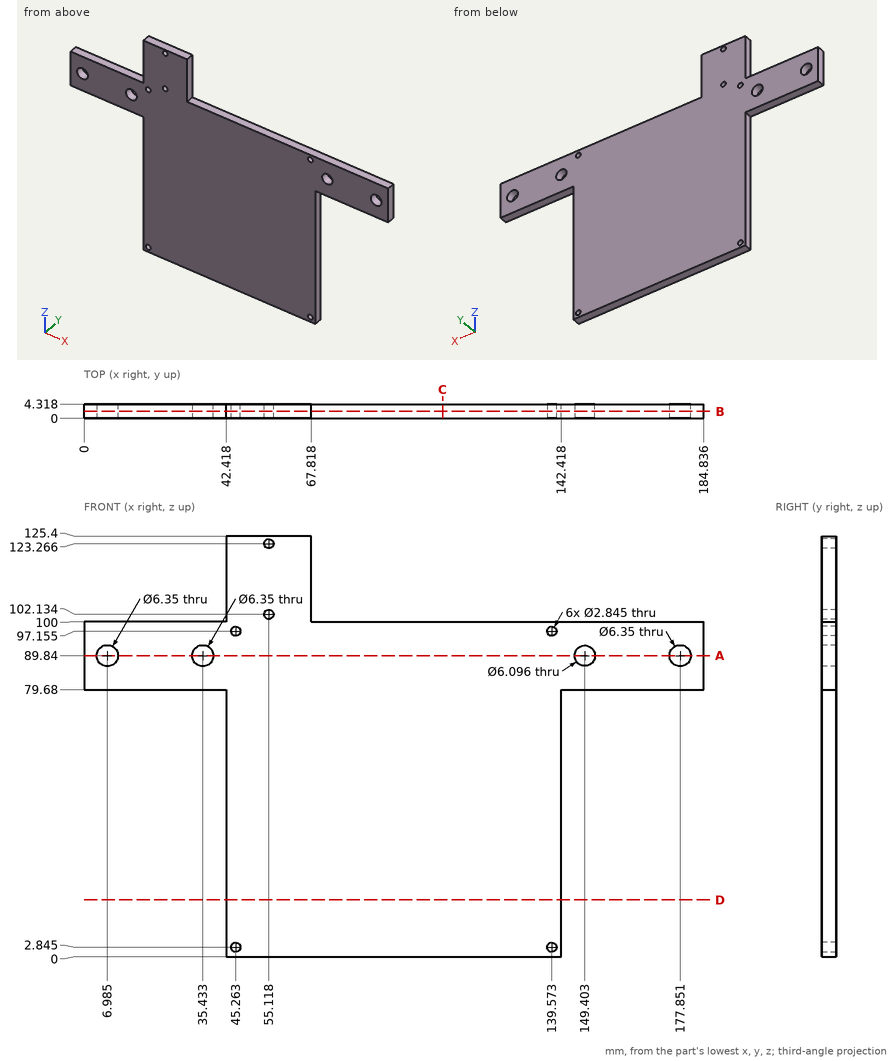
Input: dimensioned drawing with shaded views. Units: mm. Origin: part minimum x, y, z. Coordinates: 2 decimals unless noted, no trailing zeros. Write each loop counter-clockwise with the first axis right and the second up, starting at its lowest first coordinate (ties: lowest second). Pieces come first, ordered by that corner, then holes. Notation, with made-up numbers: (-24, -13) -> (-14, -13) arc R24 ccw to (-14, -1) -> close; hole circle Ø4 at (-31, -15.75). An arc over 180 degrees is marked (long way). Return JSON: item names as keys, results as strings. Group by question number.
1) Section query D-D, the plane z = 17. Return loops of the section in (x, y).
2) Section query C-C, the plane x = 107. Return loops of the section in (y, z), plus the area to 3 significant figures.
3) Section query B-B, the plane y = 2.15. State how many separate pieces and enclosed holes the cut face has, plus the area to 3 significant figures.
4) Ray query, line 1 along X through (y, z) = (3.2, 89.84) (1 decimal); line 2 along X through (y, z) = (3.3, 102) (1 decimal); line 3 along X through (y, z) = (3.95, 111). Return the intervals inside material, ascending.
5) Contact query for flat-ended pins moving along their axis: P1, Ø5.5, axis at x = 149.403, z = 89.84, coming from the -Y side; P2, Ø1.3, axis at x = 11.5, y = 3, coming from the +Z side; P3, Ø1, axis at y = 1.5, z = 51, coming from the +X side; P4, Ø1, axis at x = 38.5, y = 2, coming from the -Z side. Output: stop coordinate, or through.
6) Section query A-A, the plane z = 89.84. Return loops of the section in (x, y) (1 decimal).
From the geometry:
{
 "1": {"outline": "(42.42, 0) -> (142.42, 0) -> (142.42, 4.32) -> (42.42, 4.32) -> close"},
 "2": {"outline": "(0, 0) -> (4.32, 0) -> (4.32, 100) -> (0, 100) -> close", "area": "432 mm²"},
 "3": {"separate pieces": "1", "enclosed holes": "10", "area": "12,200 mm²"},
 "4": {"line 1": "0 to 3.8, 10.2 to 32.3, 38.6 to 146.4, 152.5 to 174.7, 181 to 184.8", "line 2": "42.4 to 53.7, 56.5 to 67.8", "line 3": "42.42 to 67.82"},
 "5": {"P1": "through", "P2": "z = 100", "P3": "x = 142.42", "P4": "z = 79.68"},
 "6": {"outline": "(0, 0) -> (3.8, 0) -> (3.8, 4.3) -> (0, 4.3) -> close; (10.2, 0) -> (32.3, 0) -> (32.3, 4.3) -> (10.2, 4.3) -> close; (38.6, 0) -> (146.4, 0) -> (146.4, 4.3) -> (38.6, 4.3) -> close; (152.5, 0) -> (174.7, 0) -> (174.7, 4.3) -> (152.5, 4.3) -> close; (181, 0) -> (184.8, 0) -> (184.8, 4.3) -> (181, 4.3) -> close"}
}
